```python
from build123d import *

# Parameters (mm, degrees)
BOSS_EXTRUDE1_DEPTH            = 50
SKETCH7_R                      = 16
CUT_EXTRUDE2_DEPTH             = 268.339938863
SKETCH8_R                      = 18.6
CUT_EXTRUDE3_DEPTH             = 9
FILLET2_R                      = 10
M5_CLEARANCE_HOLE2_D           = 5.5
M5_CLEARANCE_HOLE2_CSINK_D     = 5.55
M5_CLEARANCE_HOLE2_CSINK_ANGLE = 90
FILLET1_R                      = 10


# Read off the part's stored shape, not the designer's step: M5 Clearance Hole3
with BuildPart() as part:
    # Sketch1 → Boss-Extrude1 (new body)
    with BuildSketch(Plane(origin=(0, 0, 0), x_dir=(1, 0, 0), z_dir=(0, 1, 0))):
        Polygon((15, 15), (15, 250), (0, 250), (0, 0), (95.440306509, 0), (95.440306509, 15), align=None)
        Polygon((40.440306509, 15), (15, 99.801021696), (15, 65), (30, 15), align=None)
    extrude(amount=BOSS_EXTRUDE1_DEPTH)

    # Sketch7 → Cut-Extrude2 (cut, through all)
    with BuildSketch(Plane(origin=(15, 0, 0), x_dir=(0, 0, -1), z_dir=(1, 0, 0))):
        with Locations((210, 25)):
            Circle(SKETCH7_R)
    extrude(amount=-CUT_EXTRUDE2_DEPTH, mode=Mode.SUBTRACT)

    # Sketch8 → Cut-Extrude3 (cut)
    with BuildSketch(Plane.ZY.offset(-15)):
        with Locations((-210, 25)):
            Circle(SKETCH8_R)
    extrude(amount=CUT_EXTRUDE3_DEPTH, mode=Mode.SUBTRACT)

    # Fillet2
    fillet2_edges = [part.edges().sort_by_distance(p)[0] for p in [
        (0, 25, 0),
    ]]
    fillet(fillet2_edges, radius=FILLET2_R)

    # M5 Clearance Hole2 (through all)
    with Locations(Plane.ZY):
        with Locations((-240, 32.5), (-240, 17.5)):
            CounterSinkHole(M5_CLEARANCE_HOLE2_D / 2, M5_CLEARANCE_HOLE2_CSINK_D / 2, counter_sink_angle=M5_CLEARANCE_HOLE2_CSINK_ANGLE)

    # M5 Clearance Hole3 outline → M5 Clearance Hole3 (revolve, cut)
    with BuildSketch(Plane(origin=(55.440306509, 40, 0), x_dir=(1, 0, 0), z_dir=(0, -1, 0))):
        Polygon((2.75, -14.975), (2.75, 0), (0, 0), (0, -15), (2.775, -15), align=None)
    revolve(axis=Axis((55.440306509, 40, 0), (0, 0, 1)), mode=Mode.SUBTRACT)

    # M5 Clearance Hole3 2 outline → M5 Clearance Hole3 2 (revolve, cut)
    with BuildSketch(Plane(origin=(85.440306509, 10, 0), x_dir=(1, 0, 0), z_dir=(0, -1, 0))):
        Polygon((2.75, -14.975), (2.75, 0), (0, 0), (0, -15), (2.775, -15), align=None)
    revolve(axis=Axis((85.440306509, 10, 0), (0, 0, 1)), mode=Mode.SUBTRACT)

    # M5 Clearance Hole3 3 outline → M5 Clearance Hole3 3 (revolve, cut)
    with BuildSketch(Plane(origin=(55.440306509, 10, 0), x_dir=(1, 0, 0), z_dir=(0, -1, 0))):
        Polygon((2.75, -14.975), (2.75, 0), (0, 0), (0, -15), (2.775, -15), align=None)
    revolve(axis=Axis((55.440306509, 10, 0), (0, 0, 1)), mode=Mode.SUBTRACT)

    # M5 Clearance Hole3 4 outline → M5 Clearance Hole3 4 (revolve, cut)
    with BuildSketch(Plane(origin=(85.440306509, 40, 0), x_dir=(1, 0, 0), z_dir=(0, -1, 0))):
        Polygon((2.75, -14.975), (2.75, 0), (0, 0), (0, -15), (2.775, -15), align=None)
    revolve(axis=Axis((85.440306509, 40, 0), (0, 0, 1)), mode=Mode.SUBTRACT)

    # Fillet1
    fillet1_edges = [part.edges().sort_by_distance(p)[0] for p in [
        (95.440306509, 0, -7.5),
        (7.5, 0, -250),
        (7.5, 50, -250),
        (95.440306509, 50, -7.5),
    ]]
    fillet(fillet1_edges, radius=FILLET1_R)


solid = part.part
```
Design review of the part built by this model. Coordinates are the model's own, in mm. A direction names the side the tool comes from. Give positions to 0.01 mm unless a question says otherwise; leave off trailing zeros. Loops run counter-clockwise (first coordinate to the right, second up) from the corner with the lowest first, then second, coordinate; pieces in that order, holes last. Notation, with made-up numbers: M -31.75,43 L -1.75,43 A25 cw -1.75,56 Z; hole C 76,-8 d4. An arc over 180 degrees is marked long. Return JSON: item names as keys, results as strings. Group by question number.
Item 1: Insertion check: pin 1 Ø3.5 at (y, z) = (32.5, -240) entering from +X; pin 2 Ø1 at (x, y) = (46.5, 35) entering from -Z; pin 3 Ø18.5 at (y, z) = (16.5, -211) entering from +X; pin 4 Ø1 at (y, z) = (24, -149.5) entering from +X. Each pin has a flat end and moves straight along its axis. Give the tip position at first contact, or say it passes through.
Item 2: Tool access review of faces 4 (the cylindrical face through (10.56, 37.57, -223.71)), 5 (the flat face through (52, 25, 0)), 6 (the flat face through (15, 25, -157)): name each direction out of +Z, -Z, +X, -X, +Y, -Y from which nothing blocks a thin tool from reaching the whole face with its end or side.
Item 3: For probe 1 along Y at (x, z) = (9.25, -240); probe 2 along Z at (x, y) = (10, 32); probe 3 along Y at (x, z) = (10, -210), list the stretches that pass through material, from the lowest coordinate up.
Item 4: We need section B-B (y = 17.5). Give the boundary of the cut face in (x, z) (3 decimals), and give its area (3 significant figures).
Item 5: We need section C-C (x = 22). Give the boundary of the cut face in (y, z).
Item 6: We need section A-A (z = -210). Give the boundary of the cut face in (x, y), and give its area (3 significant figures).
Item 7: We need section D-D (z = -113). Give the boundary of the cut face in (x, y), and give its area (3 significant figures).
Item 8: Mouldability with a two-part tool opening along Y and no side actions: class faces 1 (the flat face through (6, 40.24, -204.58)), 2 (the flat face through (68, 25, -15)), 3 (the cylindrical face through (92.43, 2.85, -7.6)) as released by +Y, released by -Y, zero draft, split by the parting line, or undercut.
Output:
{
 "1": {"pin 1": "passes through", "pin 2": "stops at z = -15", "pin 3": "stops at x = 6", "pin 4": "stops at x = 15"},
 "2": {"face 4": "+X", "face 5": "+Z, +X, -X, +Y, -Y", "face 6": "-Z, +X, +Y, -Y"},
 "3": {"probe 1": "y = 0 to 14.75, 20.25 to 29.75, 35.25 to 50", "probe 2": "z = -250 to -242.7, -237.3 to -227.23, -192.77 to 0", "probe 3": "y = 0 to 6.4, 43.6 to 50"},
 "4": {"outline": "M 0,-250 L 15,-250 L 15,-242.75 L 0.025,-242.75 L 0,-242.775 Z; M 0,-237.225 L 0.025,-237.25 L 15,-237.25 L 15,-227.021 L 6,-227.021 L 6,-224.133 L 0,-224.133 Z; M 0,-195.867 L 6,-195.867 L 6,-192.979 L 15,-192.979 L 15,-99.801 L 40.44,-15 L 95.44,-15 L 95.44,0 L 10,0 A10 ccw 0,-10 Z; hole M 15,-65 L 30,-15 L 15,-15 Z", "area": "5,080 mm^2"},
 "5": {"outline": "M 0,-76.47 L 50,-76.47 L 50,-41.67 L 0,-41.67 Z; M 0,-15 L 50,-15 L 50,0 L 0,0 Z"},
 "6": {"outline": "M 0,0 L 15,0 L 15,6.4 L 6,6.4 L 6,9 L 0,9 Z; M 0,41 L 6,41 L 6,43.6 L 15,43.6 L 15,50 L 0,50 Z", "area": "223 mm^2"},
 "7": {"outline": "M 0,0 L 15,0 L 15,50 L 0,50 Z", "area": "750 mm^2"},
 "8": {"face 1": "undercut", "face 2": "zero draft", "face 3": "released by -Y"}
}
